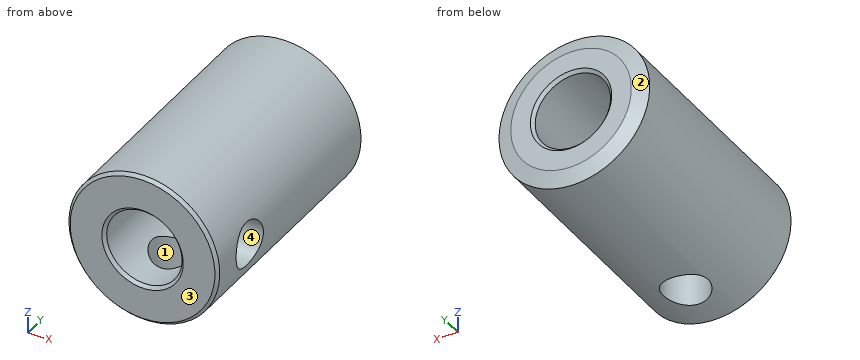
from build123d import *

# Parameters (mm, degrees)
SKETCH1_R               = 5
SKETCH1_R_2             = 2.5
BOSS_EXTRUDE1_DEPTH     = 16.1
CHAMFER1_SIZE           = 0.2
CHAMFER2_SIZE           = 1
CHAMFER2_SIZE2          = 0.363970234
CUT_EXTRUDE1_REACH      = 21.601
CUT_EXTRUDE1_END_RADIUS = 2.5
SKETCH2_R               = 1.5
CIRPATTERN1_COUNT       = 2
CIRPATTERN1_ANGLE       = 90


with BuildPart() as part:
    # Sketch1 → Boss-Extrude1 (new body)
    with BuildSketch(Plane(origin=(0, 0, 0), x_dir=(1, 0, 0), z_dir=(0, 1, 0))):
        with Locations(Location((0, 0, 0), (0, 0, 270))):
            Circle(SKETCH1_R)
        with Locations(Location((0, 0, 0), (0, 0, 270))):
            Circle(SKETCH1_R_2, mode=Mode.SUBTRACT)
    extrude(amount=BOSS_EXTRUDE1_DEPTH)

    # Chamfer1
    chamfer1_edges = [part.edges().sort_by_distance(p)[0] for p in [
        (0, 0, -5),
        (0, 0, -2.5),
        (0, 16.1, -2.5),
    ]]
    chamfer(chamfer1_edges, length=CHAMFER1_SIZE)

    # Chamfer2
    chamfer2_edges = [part.edges().sort_by_distance(p)[0] for p in [
        (0, 16.1, -5),
    ]]
    chamfer2_side = [part.faces().sort_by_distance(p)[0] for p in [
        (0, 16.1, -2.841421356),
    ]]
    chamfer(chamfer2_edges, length=CHAMFER2_SIZE, length2=CHAMFER2_SIZE2, reference=chamfer2_side[0])

    # Cut-Extrude1: up to this cylinder (the profile starts outside it)
    cut_extrude1_end = Plane(origin=(0, 3.5, 0), z_dir=(0, -1, 0)) * Cylinder(CUT_EXTRUDE1_END_RADIUS, 49.202, mode=Mode.PRIVATE)
    # Sketch2 → Cut-Extrude1 (cut, up to the surface)
    with BuildSketch(Plane(origin=(0, 0, -5), x_dir=(-1, 0, 0), z_dir=(0, 0, -1)), mode=Mode.PRIVATE) as cut_extrude1_sk1:
        with Locations((0, 3.5)):
            Circle(SKETCH2_R)
    cut_extrude1_tool1 = extrude(cut_extrude1_sk1.sketch, amount=-CUT_EXTRUDE1_REACH, mode=Mode.PRIVATE) - cut_extrude1_end
    cut_extrude1 = cut_extrude1_tool1.solids().sort_by_distance((0, 3.5, -5))[0]
    add(cut_extrude1, mode=Mode.SUBTRACT)

    # CirPattern1: Cut-Extrude1 ×2 about axis
    cirpattern1_axis = Axis((0, 15.9, 0), (0, -1, 0))
    for i in range(1, CIRPATTERN1_COUNT):
        add(cut_extrude1.rotate(cirpattern1_axis, i * CIRPATTERN1_ANGLE / (CIRPATTERN1_COUNT - 1)), mode=Mode.SUBTRACT)


solid = part.part
The listing builds one solid part. Answer for the finished solid, in the listing's coordinates (mm). Face numbers are marked on the shaded views. Give positions to 0.01 mm unless a question says otherwise; leave off trailing zeros. Loops run counter-clockwise (first coordinate to the right, second up) from the corner with the lowest first, then second, coordinate; pieces in that order, holes last. Notation, with made-up numbers: (41.5, 34) - (80.5, 34) arc R13 cw to (80.5, 55) - close; hole circle Ø3 at (-14.5, -11.5). An arc over 180 degrees is marked (long way). Use one line per item in the form item = value.
1. Find the intervals of material crossed by line 1 along Z through (x, y) = (0, 7.5); line 2 along Z through (x, y) = (0, 4.75), in increasing order. Write a range as [from, to].
Calculated:
line_1 = [-5, -2.5], [2.5, 5]
line_2 = [2.5, 5]
2. Given pin 1 Ø4 at (x, y) = (3, 10) entering from +Z; pin 2 Ø1.5 at (x, y) = (3.5, 1.5) entering from -Z; pin 3 Ø4 at (x, z) = (0, 0) entering from +Y, each flat-ended and moving along its own axis, determine where each tip first touches the part or whether it passes through.
Calculated:
pin_1 = 4.9
pin_2 = -4.18
pin_3 = through
3. Section D-D on y = 6.75 is taken. Give the vertices of the cut face in (x, z).
Calculated:
outline = circle Ø10 at (0, 0); hole circle Ø5 at (0, 0)
4. Section B-B on z = 0 is taken. Give the vertices of the cut face in (x, y).
Calculated:
outline = (-5, 0.2) - (-4.8, 0) - (-2.7, 0) - (-2.5, 0.2) - (-2.5, 15.9) - (-2.7, 16.1) - (-4, 16.1) - (-5, 15.74) - close; (2.5, 0.2) - (2.7, 0) - (4.8, 0) - (5, 0.2) - (5, 2) - (2.5, 2) - close; (2.5, 5) - (5, 5) - (5, 15.74) - (4, 16.1) - (2.7, 16.1) - (2.5, 15.9) - close
5. Section A-A on x = 0 is taken. Give the vertices of the cut face in (y, z), then the cut area to 3 significant figures.
Calculated:
outline = (0, -4.8) - (0.2, -5) - (2, -5) - (2, -2.5) - (0.2, -2.5) - (0, -2.7) - close; (0, 2.7) - (0.2, 2.5) - (15.9, 2.5) - (16.1, 2.7) - (16.1, 4) - (15.74, 5) - (0.2, 5) - (0, 4.8) - close; (5, -5) - (15.74, -5) - (16.1, -4) - (16.1, -2.7) - (15.9, -2.5) - (5, -2.5) - close
area = 72.5 mm^2
6. The mould has two halves that part along Y. Classify the marked faces 1, 2, 3 and 4: pulls with the +Y half, pulls with the -Y half, needs draft (parallel to the pull), parting line crosses it, or undercut.
Calculated:
face_1 = undercut
face_2 = pulls with the +Y half
face_3 = pulls with the -Y half
face_4 = undercut
7. Section C-C on y = 3.5 is taken. Give the vertices of the cut face in (x, z), then the cut area to 3 significant figures.
Calculated:
outline = (-1.5, -4.77) - (-1.5, -2) arc R2.5 cw (long way) to (2, 1.5) - (4.77, 1.5) arc R5 ccw (long way) to start; (1.5, -4.77) arc R5 ccw to (4.77, -1.5) - (2, -1.5) arc R2.5 cw to (1.5, -2) - close
area = 43.4 mm^2
